Verification items for this drawing (mm, ordinates from the low corner). Coordinates: 2 decimals unless noted, no trailing zeros. Write each loop counter-clockwise with the first axis right and the second up, starting at its lowest first coordinate (ties: lowest second). Pieces come first, ordered by that corner, then holes. Notation, with made-up numbers: M 26,-34.5 L 73,-34.5 A14 cw 73,-22.5 Z; hole C -8,50.25 d8. An arc over 180 degrees is marked long. Put each result on its own line as item: value. Start each with the question number.
1) Mould release check, pull along X, two halves, no side actions. Record for the marked faces 1, 2 and 3: released by +X, released by -X, zero draft, split by the parting line, or undercut.
2) Cross-section at B-B on x = 36.5. Record the cut outline in (y, z).
3) Cross-section at A-A on y = 94. Record the cut outline in (x, z), plus the area to 3 significant figures.
4) Scan lines: line 1 along Z through (x, y) = (16.5, 7.5); line 2 along Y through (x, z) = (52.5, 7.5) (1 decimal). Record each from-to range of solid material in increasing order.
5) Gauge pin test, flat end, axial feed: pin 1 (1.5 mm diameter, centred on x = 13, y = 23, fed in from +Z). Record the tip position at first contact, or that the pin passes through.
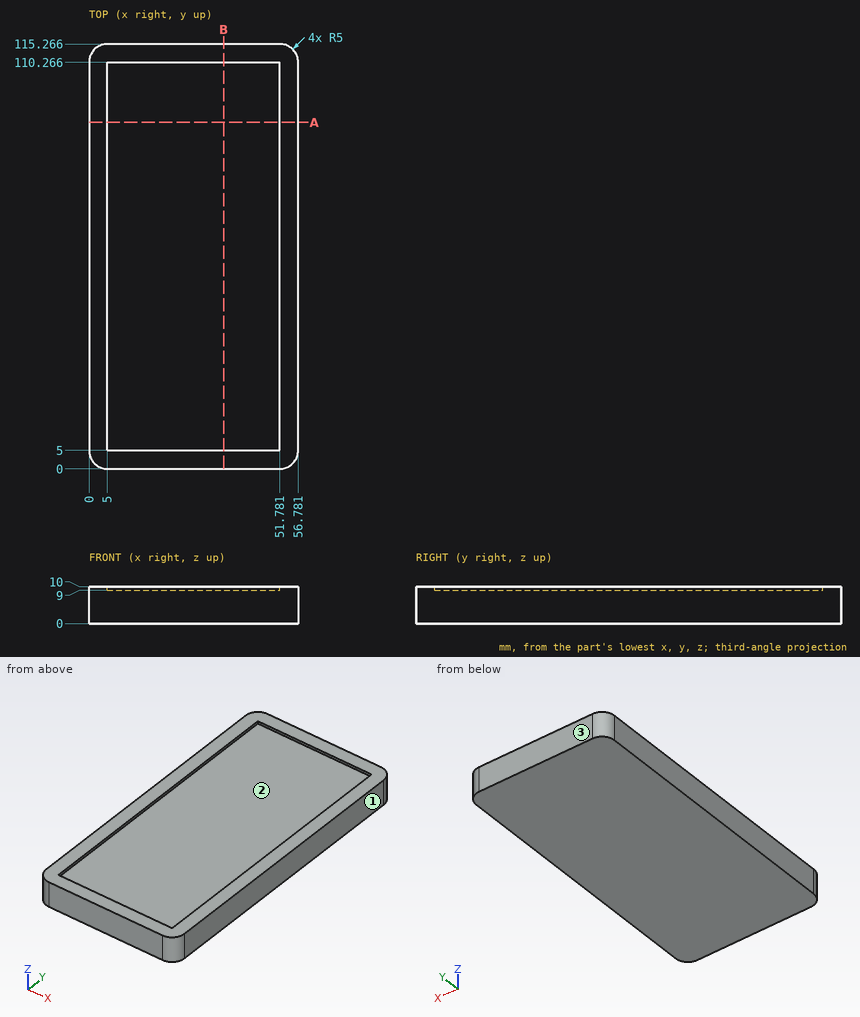
Answer key:
1. face 1: released by +X
1. face 2: undercut
1. face 3: zero draft
2. outline: M 0,0 L 115.27,0 L 115.27,10 L 110.27,10 L 110.27,9 L 5,9 L 5,10 L 0,10 Z
3. outline: M 0,0 L 56.78,0 L 56.78,10 L 51.78,10 L 51.78,9 L 5,9 L 5,10 L 0,10 Z
3. area: 521 mm²
4. line 1: z = 0 to 9
4. line 2: y = 0.1 to 115.2
5. pin 1: stops at z = 9
